For this review, take the finished solid that the model builds, in its own axes (mm). A direction names the side the tool comes from. Round coordinates to 2 decimals unless told otherwise and drop trailing zeros. Write each loop counter-clockwise with the first axis right and the second up, starting at its lowest first coordinate (ties: lowest second). Pieces come first, ordered by that corner, then holes.
from build123d import *

# Parameters (mm, degrees)
SKETCH1_W               = 50.8
SKETCH1_H               = 527.05
BOSS_EXTRUDE1_DEPTH     = 12.7
SHELL1_T                = -1.5875
CUT_EXTRUDE1_DEPTH      = 266.050703876
CUT_EXTRUDE1_DEPTH_BACK = 266.050703876
SKETCH2_R               = 2.4892
CUT_EXTRUDE2_DEPTH      = 266.050703876
CUT_EXTRUDE2_DEPTH_BACK = 266.050703876
SKETCH3_R               = 2.4892


with BuildPart() as part:
    # Sketch1 → Boss-Extrude1 (new, symmetric)
    with BuildSketch(Plane.XY):
        Rectangle(SKETCH1_W, SKETCH1_H)
    extrude(amount=BOSS_EXTRUDE1_DEPTH, both=True)

    # Shell1
    shell1_openings = [part.faces().sort_by_distance(p)[0] for p in [
        (0, -263.525, 0),
        (0, 263.525, 0),
    ]]
    offset(amount=SHELL1_T, openings=shell1_openings, kind=Kind.INTERSECTION)

    # Sketch2 → Cut-Extrude1 (cut, two sides: drawn at the far end of the back side and taken through both)
    with BuildSketch(Plane.XY.offset(-CUT_EXTRUDE1_DEPTH_BACK)):
        with Locations((-12.7, -250.825)):
            Circle(SKETCH2_R)
        with Locations((12.7, -250.825)):
            Circle(SKETCH2_R)
        with Locations(Location((12.7, 250.825, 0), (0, 0, 180))):
            Circle(SKETCH2_R)
        with Locations(Location((-12.7, 250.825, 0), (0, 0, 180))):
            Circle(SKETCH2_R)
    extrude(amount=CUT_EXTRUDE1_DEPTH + CUT_EXTRUDE1_DEPTH_BACK, mode=Mode.SUBTRACT)

    # Sketch3 → Cut-Extrude2 (cut, two sides: drawn at the far end of the back side and taken through both)
    with BuildSketch(Plane(origin=(0, 0, 0), x_dir=(0, 0, -1), z_dir=(1, 0, 0)).offset(-CUT_EXTRUDE2_DEPTH_BACK)):
        with Locations((0, -250.825)):
            Circle(SKETCH3_R)
        with Locations((0, 250.825)):
            Circle(SKETCH3_R)
    extrude(amount=CUT_EXTRUDE2_DEPTH + CUT_EXTRUDE2_DEPTH_BACK, mode=Mode.SUBTRACT)


solid = part.part
(1) We need section B-B, the plane x = -4.5. Give the boundary of the cut face in (y, z) (1 decimal).
Geometry check:
outline: (-263.5, -12.7) - (263.5, -12.7) - (263.5, -11.1) - (-263.5, -11.1) - close; (-263.5, 11.1) - (263.5, 11.1) - (263.5, 12.7) - (-263.5, 12.7) - close
(2) For line 1 along Y through (x, z) = (-24.85, 0) (3 decimals); line 2 along X through (y, z) = (-162, -1); line 3 along Z through (x, y) = (16.5, -35.5), list the stretches that pass through material, from the lowest coordinate up.
Geometry check:
line 1: y = -263.525 to -253.314, -248.336 to 248.336, 253.314 to 263.525
line 2: x = -25.4 to -23.81, 23.81 to 25.4
line 3: z = -12.7 to -11.11, 11.11 to 12.7
(3) We need section C-C, the plane y = -104. Give the boundary of the cut face in (x, z).
Geometry check:
outline: (-25.4, -12.7) - (25.4, -12.7) - (25.4, 12.7) - (-25.4, 12.7) - close; hole (-23.81, -11.11) - (23.81, -11.11) - (23.81, 11.11) - (-23.81, 11.11) - close
(4) We need section A-A, the plane z = 6.75. Give the boundary of the cut face in (x, y) (1 decimal), and give its area (3 significant figures).
Geometry check:
outline: (-25.4, -263.5) - (-23.8, -263.5) - (-23.8, 263.5) - (-25.4, 263.5) - close; (23.8, -263.5) - (25.4, -263.5) - (25.4, 263.5) - (23.8, 263.5) - close
area: 1,670 mm2
(5) For faces 4 (the face through (0, 263.525, -12)), 5 (the face through (-23.812, -4, 0)), list the 3-axis set-ups (+Z, -Z, +X, -X, +Y, -Y) from which the entire face can be reached by the end or side of a thin tool; tool diameter is ignored.
Geometry check:
face 4: +Z, -Z, +X, -X, +Y
face 5: +Y, -Y
(6) For pin 1 Ø6.5 at (x, y) = (-12.7, 250.825) entering from +Z, flat-tipped, find the tip position at first contact; note if it passes through.
Geometry check:
pin 1: stops at z = 12.7
(7) Mouldability with a two-part tool opening along Z and no side actions: class faces 1 (the face through (0, 4, -12.7)), 2 (the face through (23.812, -4, 0)), 3 (the face through (-25.4, -4, 0)) as pulls with the +Z half, pulls with the -Z half, needs draft (parallel to the pull), parting line crosses it, or undercut.
Geometry check:
face 1: pulls with the -Z half
face 2: undercut
face 3: needs draft
